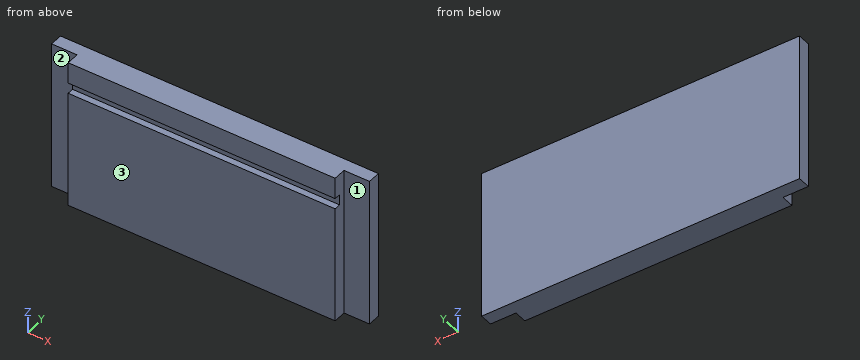
```python
from build123d import *

# Parameters (mm, degrees)
F1_DEPTH = 150
F2_W     = 12
F2_H     = 70
F3_DEPTH = 6


# Not quite as in the source:
# - a feature names something its author has since deleted; it is built from what else it names


with BuildPart() as f1:
    # F0 (on Right) → F1 (new body)
    with BuildSketch(Plane.YZ):
        Polygon((-12, 0), (0, 0), (0, 70), (-12, 70), (-12, 60), (-9, 60), (-9, 55), (-12, 55), align=None)
    extrude(amount=F1_DEPTH)

    # F2 (on face) → F3 (cut)
    with BuildSketch(Plane.XZ.offset(12)):
        with Locations((144, 35)):
            Rectangle(F2_W, F2_H)
        with Locations((6, 35)):
            Rectangle(F2_W, F2_H)
    extrude(amount=-F3_DEPTH, mode=Mode.SUBTRACT)


solid = f1.part
```
Verification items for the finished model (mm, model axes). Face numbers are marked on the shaded views. A direction names the side the tool comes from. Coordinates: 2 decimals unless noted, no trailing zeros. Write each loop counter-clockwise with the first axis right and the second up, starting at its lowest first coordinate (ties: lowest second). Pieces come first, ordered by that corner, then holes. Notation, with made-up numbers: M 35,-12 L 57,-12 A18 ccw 57,4 Z; hole C 27,42 d3. An arc over 180 degrees is marked long. Answer as a JSON object with one key per item and string values. Group by question number.
(1) Cross-section at A-A, the plane z = 50. Record the cut outline in (x, y), and give its area (3 significant figures).
(2) Gauge pin test, flat ends, axial feed: pin 1 (3 mm diameter, centred on y = -10, z = 17.5, fed in from +X); pin 2 (1.5 mm diameter, centred on x = 83.5, z = 56.5, fed in from -Y); pin 3 (1.8 mm diameter, centred on y = -9.5, z = 22.5, fed in from -X). Record the tip position at first contact, or that the pin passes through.
(3) Material ranges on line 1 (Z direction, x = 84, y = -11.5); line 2 (X direction, y = -7.5, z = 31); line 3 (Y direction, x = 8, z = 5), recorded low to high.
(4) Tool access check on the marked faces 1, 2 and 3. Record the directions out of +Z, -Z, +X, -X, +Y, -Y that give a thin tool (end or side, any length) a straight path to the whole face; none if there is none.
(5) Cross-section at B-B, the plane x = 99. Record the cut outline in (y, z).
Reply:
{
 "1": {"outline": "M 0,-6 L 12,-6 L 12,-12 L 138,-12 L 138,-6 L 150,-6 L 150,0 L 0,0 Z", "area": "1,660 mm²"},
 "2": {"pin 1": "x = 138", "pin 2": "y = -9", "pin 3": "x = 12"},
 "3": {"line 1": "0 to 55, 60 to 70", "line 2": "12 to 138", "line 3": "-6 to 0"},
 "4": {"face 1": "+Z, -Z, +X, -Y", "face 2": "+Z, -Z, -X, -Y", "face 3": "+Z, -Z, +X, -X, -Y"},
 "5": {"outline": "M -12,0 L 0,0 L 0,70 L -12,70 L -12,60 L -9,60 L -9,55 L -12,55 Z"}
}
